Design review of the part built by this model. Coordinates are the model's own, in mm. Face numbers are marked on the shaded views. Give positions to 0.01 mm unless a question says otherwise; leave off trailing zeros. Loops run counter-clockwise (first coordinate to the right, second up) from the corner with the lowest first, then second, coordinate; pieces in that order, holes last. Notation, with made-up numbers: (-11, -34.5) -> (-2, -34.5) arc R20 ccw to (-2, -2.5) -> close; hole circle Ø1 at (36, 38). An arc over 180 degrees is marked (long way). Use CSV: the item, a comma, the result in double quotes. Start each with the question number.
Item 1: We need section A-A (x = 8.5). State the section outline as (y, z) points, plus the area to 3 significant figures.
Item 2: Clearance check with a flat-ended pin moving along its axis: pin 1 (7.5 mm diameter, centred on x = 13, y = 13.5, fed in from +Z). State where the tip first meets the part, or that it passes through.
Item 3: The part is to be moulded in two halves that separate along X. For the marked faces 1 and 2, say which applies: +X half, -X half, draft (parallel to the pull), parting line (faces both ways), or undercut.
Item 4: Wall thickness on line 1 along X through (y, z) = (13, 2.4); line 2 along Y through (x, z) = (24.5, 1.9); line 3 along Z through (x, y) = (24, 23): over which ranges is each line inside the solid? List them lowest first. Write a range as from..to.
Item 5: We need section B-B (y = 6). State the section outline as (x, z) points.
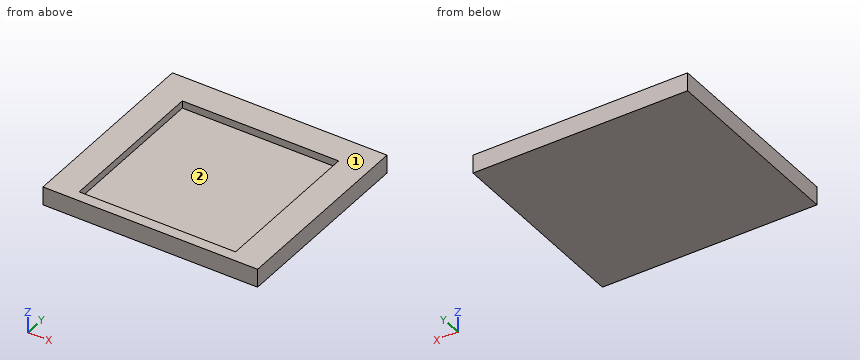
from build123d import *

# Parameters (mm, degrees)
SKETCH1_W           = 35
SKETCH1_H           = 35
BOSS_EXTRUDE1_DEPTH = 3
SKETCH2_W           = 25.5
SKETCH2_H           = 25.5
CUT_EXTRUDE1_DEPTH  = 1.2
SKETCH3_W           = 35
SKETCH3_H           = 3
CUT_EXTRUDE2_DEPTH  = 3


with BuildPart() as part:
    # Sketch1 → Boss-Extrude1 (new body)
    with BuildSketch(Plane.XY):
        with Locations((17.5, 17.5)):
            Rectangle(SKETCH1_W, SKETCH1_H)
    extrude(amount=BOSS_EXTRUDE1_DEPTH)

    # Sketch2 → Cut-Extrude1 (cut)
    with BuildSketch(Plane.XY.offset(3)):
        with Locations((17.5, 17.5)):
            Rectangle(SKETCH2_W, SKETCH2_H)
    extrude(amount=-CUT_EXTRUDE1_DEPTH, mode=Mode.SUBTRACT)

    # Sketch3 → Cut-Extrude2 (cut)
    with BuildSketch(Plane.XZ):
        with Locations((17.5, 1.5)):
            Rectangle(SKETCH3_W, SKETCH3_H)
    extrude(amount=-CUT_EXTRUDE2_DEPTH, mode=Mode.SUBTRACT)


solid = part.part
Results found:
1,outline,"(3, 0) -> (35, 0) -> (35, 3) -> (30.25, 3) -> (30.25, 1.8) -> (4.75, 1.8) -> (4.75, 3) -> (3, 3) -> close"
1,area,"65.4 mm²"
2,pin 1,"z = 1.8"
3,face 1,"draft"
3,face 2,"undercut"
4,line 1,"0..4.75, 30.25..35"
4,line 2,"3..4.75, 30.25..35"
4,line 3,"0..1.8"
5,outline,"(0, 0) -> (35, 0) -> (35, 3) -> (30.25, 3) -> (30.25, 1.8) -> (4.75, 1.8) -> (4.75, 3) -> (0, 3) -> close"
